```python
from build123d import *

# Parameters (mm, degrees)
SKETCH1_W           = 176
SKETCH1_H           = 103
SKETCH1_W_2         = 166
SKETCH1_H_2         = 93
BOSS_EXTRUDE1_DEPTH = 160
CUT_EXTRUDE1_REACH  = 261.201
SKETCH2_W           = 166
SKETCH2_H           = 5


with BuildPart() as part:
    # Sketch1 → Boss-Extrude1 (new body)
    with BuildSketch(Plane(origin=(0, 0, 0), x_dir=(1, 0, 0), z_dir=(0, 1, 0))):
        with Locations((88, 51.5)):
            Rectangle(SKETCH1_W, SKETCH1_H)
        with Locations((88, 51.5)):
            Rectangle(SKETCH1_W_2, SKETCH1_H_2, mode=Mode.SUBTRACT)
    extrude(amount=BOSS_EXTRUDE1_DEPTH)

    # Sketch2 → Cut-Extrude1 (cut, up to next)
    with BuildSketch(Plane.XY, mode=Mode.PRIVATE) as cut_extrude1_sk1:
        with Locations((88, 2.5)):
            Rectangle(SKETCH2_W, SKETCH2_H)
    cut_extrude1_tool1 = extrude(cut_extrude1_sk1.sketch, amount=-CUT_EXTRUDE1_REACH, mode=Mode.PRIVATE) & part.part
    add(cut_extrude1_tool1.solids().sort_by_distance((88, 2.5, 0))[0], mode=Mode.SUBTRACT)


solid = part.part
```
Work out the finished part from the listing and answer in its coordinate system (mm). A direction names the side the tool comes from. Round coordinates to 2 decimals unless told otherwise and drop trailing zeros. Write each loop counter-clockwise with the first axis right and the second up, starting at its lowest first coordinate (ties: lowest second). Pieces come first, ordered by that corner, then holes.
1) Which of the six approach directions +Z, -Z, +X, -X, +Y, -Y give full straight-line access (tool end or side, diameter ignored) to faces 4 (the face through (87, 5, -2)), 5 (the face through (88, 0, -101)), 6 (the face through (87, 79, -98))?
2) A cutting plane is placed at C-C on x = 78.5. Determine the outline of the cut face in (y, z), and give its area (4 significant figures).
3) A cutting plane is placed at A-A on y = 15. Determine the outline of the cut face in (x, z).
4) A flat-ended cylindrical pin translates along its axis: P1, Ø2.5, axis at x = 126, z = -2, coming from the -Y side. Find the tip coordinate at first contact, or state that the pin passes through.
5) A cutting plane is placed at B-B on z = -42.5. Determine the outline of the cut face in (x, y), and give its area (3 significant figures).
6) Consider probe 1 along X at (y, z) = (128, -60); probe 2 along Z at (x, y) = (73.5, 79.5). Determine where each line is inside the solid, lowest interval first.
7) Determine the mould class of faces 1 (the face through (176, 79, -51)), 2 (the face through (171, 79, -48)), 3 (the face through (87, 79, -103)) for opening direction X: pulls with the +X half, pulls with the -X half, needs draft (parallel to the pull), parting line crosses it, or undercut.
Entries:
1. face 4: +Z, -Y
1. face 5: +Z, -Z, +X, -X, -Y
1. face 6: +Y, -Y
2. outline: (0, -103) - (160, -103) - (160, -98) - (0, -98) - close; (5, -5) - (160, -5) - (160, 0) - (5, 0) - close
2. area: 1,575 mm2
3. outline: (0, -103) - (176, -103) - (176, 0) - (0, 0) - close; hole (5, -98) - (171, -98) - (171, -5) - (5, -5) - close
4. P1: stops at y = 5
5. outline: (0, 0) - (5, 0) - (5, 160) - (0, 160) - close; (171, 0) - (176, 0) - (176, 160) - (171, 160) - close
5. area: 1,600 mm2
6. probe 1: x = 0 to 5, 171 to 176
6. probe 2: z = -103 to -98, -5 to 0
7. face 1: pulls with the +X half
7. face 2: undercut
7. face 3: needs draft
